```python
from build123d import *

# Parameters (mm, degrees)
F0_W     = 25.4
F0_H     = 25.4
F1_DEPTH = 50.8
F2_R     = 4.292472
F3_R     = 10.181581
F4_DEPTH = 25.4


with BuildPart() as f1:
    # F0 (on Top) → F1 (new body)
    with BuildSketch(Plane.XY):
        Rectangle(F0_W, F0_H)
    extrude(amount=F1_DEPTH)

    # F2
    f2_edges = [f1.edges().sort_by_distance(p)[0] for p in [
        (12.7, -12.7, 25.4),
        (12.7, 12.7, 25.4),
        (-12.7, -12.7, 25.4),
        (-12.7, 12.7, 25.4),
        (0, 12.7, 0),
        (-12.7, 0, 0),
        (0, -12.7, 0),
        (12.7, 0, 0),
    ]]
    fillet(f2_edges, radius=F2_R)

    # F3 (on face) → F4 (join)
    with BuildSketch(Plane.XY.offset(50.8)):
        Circle(F3_R)
    extrude(amount=F4_DEPTH)


solid = f1.part
```
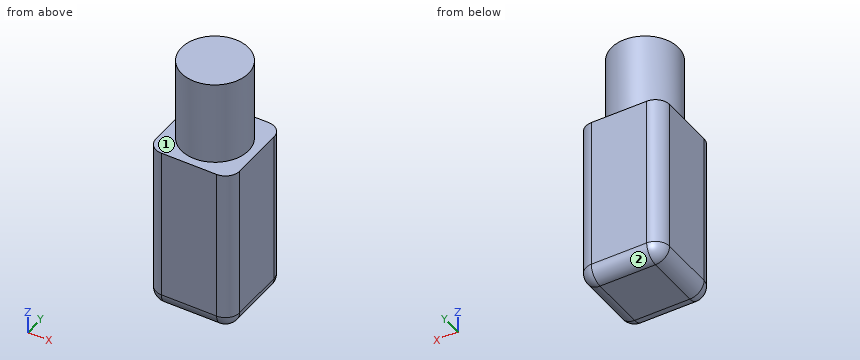
Part model, mm, in its own coordinate system. Face numbers are marked on the shaded views. A direction names the side the tool comes from. Round coordinates to 2 decimals unless told otherwise and drop trailing zeros. Loops run counter-clockwise (first coordinate to the right, second up) from the corner with the lowest first, then second, coordinate; pieces in that order, holes last.
1. Slice it at C-C (x = -5.5). Give the cut face in (y, z), and give its area (3 significant figures).
Solutions:
outline: (-12.7, 4.29) arc R4.29 ccw to (-8.41, 0) - (8.41, 0) arc R4.29 ccw to (12.7, 4.29) - (12.7, 50.8) - (8.57, 50.8) - (8.57, 76.2) - (-8.57, 76.2) - (-8.57, 50.8) - (-12.7, 50.8) - close
area: 1,720 mm2
2. Slice it at B-B (y = 0). Give the cut face in (x, z), and give its area (3 significant figures).
Solutions:
outline: (-12.7, 4.29) arc R4.29 ccw to (-8.41, 0) - (8.41, 0) arc R4.29 ccw to (12.7, 4.29) - (12.7, 50.8) - (10.18, 50.8) - (10.18, 76.2) - (-10.18, 76.2) - (-10.18, 50.8) - (-12.7, 50.8) - close
area: 1,800 mm2
3. 3-axis set-ups, long thin cutter, end or side, ignore diameter. For the marked faces 1 and 2: which of +Z, -Z, +X, -X, +Y, -Y reach the whole face in a straight line?
Solutions:
face 1: +Z
face 2: -Z, +X, -X, +Y
4. Slice it at D-D (x = 11.25). Give the cut face in (y, z).
Solutions:
outline: (-11.62, 4.29) arc R3.22 ccw to (-8.41, 1.08) - (8.41, 1.08) arc R3.22 ccw to (11.62, 4.29) - (11.62, 50.8) - (-11.62, 50.8) - close
5. Slice it at A-A (z = 46). Give the cut face in (x, y).
Solutions:
outline: (-12.7, -8.41) arc R4.29 ccw to (-8.41, -12.7) - (8.41, -12.7) arc R4.29 ccw to (12.7, -8.41) - (12.7, 8.41) arc R4.29 ccw to (8.41, 12.7) - (-8.41, 12.7) arc R4.29 ccw to (-12.7, 8.41) - close
6. Drill centre lines: line 1 along Z through (x, y) = (1.75, -11.25); line 2 along Y through (x, z) = (-8, 58); line 3 along Z through (x, y) = (-9, -2.75). Where is each one in solid material? Low to high.
Solutions:
line 1: z = 1.08 to 50.8
line 2: y = -6.3 to 6.3
line 3: z = 0.04 to 76.2
7. Flat gauge pins, fed straight in: pin 1 (5 mm diameter, centred on x = -7.5, z = 52, fed in from +Y); pin 2 (1 mm diameter, centred on y = -3, z = 60.5, fed in from -X). Where does each tip first touch, or does it go through?
Solutions:
pin 1: stops at y = 12.7
pin 2: stops at x = -9.87
